from build123d import *

# Parameters (mm, degrees)
EXTRUDE_1_DEPTH     = 380
CUT_EXTRUDE_1_DEPTH = 473.016948848


with BuildPart() as part:
    # 草图2 → 凸台-拉伸1 (new body)
    with BuildSketch(Plane.XY):
        Polygon((0, 0), (-253.76618037, -118.333113287), (26.23381963, -118.333113287), (26.23381963, -108.333113287), (-208.659095334, -108.333113287), (23.662015832, 0), align=None)
    extrude(amount=EXTRUDE_1_DEPTH)

    # 草图3 → 切除-拉伸1 (cut, through all)
    with BuildSketch(Plane.XY.offset(380)):
        Polygon((-232.321111165, -108.333113287), (-253.76618037, -118.333113287), (-232.321111165, -118.333113287), align=None)
    extrude(amount=-CUT_EXTRUDE_1_DEPTH, mode=Mode.SUBTRACT)


solid = part.part
Could you check a few things on this model? Use its own coordinates, in mm. A direction names the side the tool comes from. Coordinates: 2 decimals unless noted, no trailing zeros. Loops run counter-clockwise (first coordinate to the right, second up) from the corner with the lowest first, then second, coordinate; pieces in that order, holes last. Notation, with made-up numbers: (4, 43) -> (19, 43) arc R35 ccw to (19, 80) -> close; hole circle Ø2 at (-34.5, -36.75). An arc over 180 degrees is marked (long way). Answer in a Markdown table with one row per item.
(1) Will these pins go through, and if not, where does the flat tip stop? pin 1 Ø3 at (x, z) = (-78, 217) entering from +Y; pin 2 Ø3 at (x, z) = (-201.5, 297.5) entering from +Y; pin 3 Ø8 at (y, z) = (-86, 239.5) entering from +X.
Results found:
| item | result |
|---|---|
| pin 1 | stops at y = -35.67 |
| pin 2 | stops at y = -93.26 |
| pin 3 | stops at x = -152.19 |
(2) For faces 1 (the face through (-94.125, -54.925, 187.34)), 2 (the face through (-232.321, -113, 193)), which set-ups out of +Z, -Z, +X, -X, +Y, -Y let a thin tool reach every point of the face, with its end or its side?
Results found:
| item | result |
|---|---|
| face 1 | +Z, -Z, +X |
| face 2 | +Z, -Z, -X, +Y, -Y |
(3) Thinking about a two-plate mould opening in Y: for faces 3 (the face through (26.234, -113, 187)), 4 (the face through (-90, -108.333, 187)), 5 (the face through (-105, -118.333, 187)), 6 (the face through (-114.534, -53.408, 187.34)), which applies, released by +Y, released by -Y, zero draft, split by the parting line, or undercut?
Results found:
| item | result |
|---|---|
| face 3 | zero draft |
| face 4 | undercut |
| face 5 | released by -Y |
| face 6 | released by +Y |
(4) Imagine slicing it at D-D (y = -65.5). List the corners of the cut face in (x, z) for me, plus the area to 3 significant figures.
Results found:
| item | result |
|---|---|
| outline | (-140.47, 0) -> (-116.8, 0) -> (-116.8, 380) -> (-140.47, 380) -> close |
| area | 8,990 mm^2 |
(5) Imagine slicing it at C-C (x = -217). List the corners of the cut face in (y, z) for me, plus the area to 3 significant figures.
Results found:
| item | result |
|---|---|
| outline | (-118.33, 0) -> (-101.19, 0) -> (-101.19, 380) -> (-118.33, 380) -> close |
| area | 6,510 mm^2 |
(6) Imagine slicing it at A-A (x = -186.5). List the corners of the cut face in (y, z) for me.
Results found:
| item | result |
|---|---|
| outline | (-118.33, 0) -> (-108.33, 0) -> (-108.33, 380) -> (-118.33, 380) -> close; (-98, 0) -> (-86.97, 0) -> (-86.97, 380) -> (-98, 380) -> close |
(7) Imagine slicing it at B-B (z = 63.5). List the corners of the cut face in (x, y) for me, plus the area to 3 significant figures.
Results found:
| item | result |
|---|---|
| outline | (-232.32, -118.33) -> (26.23, -118.33) -> (26.23, -108.33) -> (-208.66, -108.33) -> (23.66, 0) -> (0, 0) -> (-232.32, -108.33) -> close |
| area | 5,150 mm^2 |
(8) If I drill on probe 1 along Y at (x, z) = (-9, 157.5); probe 2 along Y at (x, z) = (-159, 364.5); probe 3 along X at (y, z) = (-39, 205.5), over which ranges is the centre line in solid material (lowest first)?
Results found:
| item | result |
|---|---|
| probe 1 | y = -118.33 to -108.33, -15.23 to -4.2 |
| probe 2 | y = -118.33 to -108.33, -85.18 to -74.14 |
| probe 3 | x = -83.64 to -59.97 |
